The model under review builds one solid part; all positions refer to its coordinate system, in mm. Face numbers are marked on the shaded views. A direction names the side the tool comes from. Give positions to 0.01 mm unless a question says otherwise; leave off trailing zeros. Loops run counter-clockwise (first coordinate to the right, second up) from the corner with the lowest first, then second, coordinate; pieces in that order, holes last. Notation, with made-up numbers: M 64.5,0.5 L 120.5,0.5 A19 cw 120.5,19.5 Z; hole C 22,30 d10. An arc over 180 degrees is marked long. Return JSON: item names as keys, results as strings.
```python
from build123d import *

# Parameters (mm, degrees)
F1_DEPTH = 76.2
F2_W     = 36.258861
F2_H     = 54.309234
F3_DEPTH = 25.4
F4_SIZE  = 5.08
F5_R     = 5.08


with BuildPart() as f1:
    # F0 (on Top) → F1 (new body)
    with BuildSketch(Plane.XY):
        Polygon((29.875379, 7.188763), (-76.368935, 7.188763), (-76.182216, -46.026755), (29.875379, -46.026755), align=None)
    extrude(amount=F1_DEPTH)

    # F2 (on face) → F3 (join)
    with BuildSketch(Plane(origin=(0, 7.188763, 0), x_dir=(-1, 0, 0), z_dir=(0, 1, 0))):
        with Locations((58.239504, 27.154617)):
            Rectangle(F2_W, F2_H)
    extrude(amount=F3_DEPTH)

    # F4
    f4_edges = [f1.edges().sort_by_distance(p)[0] for p in [
        (-76.368935, 32.588763, 27.154617),
    ]]
    chamfer(f4_edges, length=F4_SIZE)

    # F5
    f5_edges = [f1.edges().sort_by_distance(p)[0] for p in [
        (-23.246778, 7.188763, 76.2),
    ]]
    fillet(f5_edges, radius=F5_R)


solid = f1.part
```
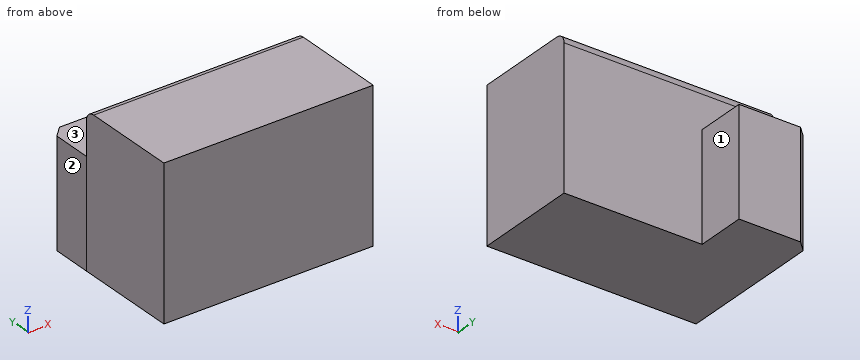
1) Wall thickness on L1, parallel to Y at x = 9, z = 16.5; L2, parallel to X at y = -1.5, z = 28; L3, parallel to X at y = 14, z = 40: over which ranges is each line inside the solid? List them lowest first. Write a range as from..to.
From the geometry:
{"L1": "-46.03..7.19", "L2": "-76.34..29.88", "L3": "-76.37..-40.11"}
2) Consider section A-A on x = -70. Write out the cut boundary in (y, z).
From the geometry:
{"outline": "M -46.03,0 L 32.59,0 L 32.59,54.31 L 7.19,54.31 L 7.19,71.12 A5.08 ccw 2.11,76.2 L -46.03,76.2 Z"}
3) Consider section C-C on y = 13. Write out the cut boundary in (x, z).
From the geometry:
{"outline": "M -76.37,0 L -40.11,0 L -40.11,54.31 L -76.37,54.31 Z"}
4) Consider section D-D on x = 9. Write out the cut boundary in (y, z).
From the geometry:
{"outline": "M -46.03,0 L 7.19,0 L 7.19,71.12 A5.08 ccw 2.11,76.2 L -46.03,76.2 Z"}
5) Tool access review of the marked faces 1, 2 and 3: name each direction out of +Z, -Z, +X, -X, +Y, -Y from which nothing blocks a thin tool from reaching the whole face with its end or side.
From the geometry:
{"face 1": "+Z, -Z, +X, +Y", "face 2": "+Z, -Z, -X, +Y, -Y", "face 3": "+Z, +X, -X, +Y"}
6) Insertion check: pin 1 (6 mm diameter, centred on x = -11, z = 9, fed in from +Y); pin 2 (12 mm diameter, centred on y = -27, z = 50, fed in from -X); pin 3 (12.5 mm diameter, centred on x = -53, y = 24.5, fed in from +Z); pin 4 (3 mm diameter, centred on x = -41.5, y = 1, fed in from -Z). Each pin has a flat end and moves straight along its axis. Give the tip position at first contact, or say it passes through.
From the geometry:
{"pin 1": "y = 7.19", "pin 2": "x = -76.27", "pin 3": "z = 54.31", "pin 4": "z = 0"}
7) Consider section B-B on z = 23. Write out the cut boundary in (x, y), then the cut area to 3 significant figures.
From the geometry:
{"outline": "M -76.37,7.19 L -76.18,-46.03 L 29.88,-46.03 L 29.88,7.19 L -40.11,7.19 L -40.11,32.59 L -71.29,32.59 L -76.37,27.51 Z", "area": "6,560 mm²"}
